Build history of the part. All positions in model axes, mm. A direction names the side the tool comes from. Give positions to 0.01 mm unless a question says otherwise; leave off trailing zeros. Loops run counter-clockwise (first coordinate to the right, second up) from the corner with the lowest first, then second, coordinate; pieces in that order, holes last. Notation, with made-up numbers: (6, 45.25) -> (20, 45.25) arc R36 ccw to (20, 80.25) -> close; hole circle Ø3 at (79.25, 22.25). An arc over 180 degrees is marked (long way). One line per question, with ' | ' between items. Start each with the question number.
(1) 3-axis set-ups, long thin cutter, end or side, ignore diameter. For faces 4 (the face through (92.284, 68.059, 113.109)), 5 (the face through (33.459, 79.964, 195.719)), 6 (the face through (105.51, 15.34, 49.21)): which of +Z, -Z, +X, -X, +Y, -Y reach the whole face in a straight line?
(2) Slice it at A-A, the plane z = 120.65. Write the cut outline in (x, y), then the cut area to 3 significant figures.
(3) Slice it at C-C, the plane z = 41.5. Write the cut outline in (x, y).
(4) Mould opens along X. For faces 1 (the face through (70.713, 79.585, 68.393)), 2 (the face through (-5.603, 19, 79)), 3 (the face through (104.887, 19, 79)) say: pulls with the +X half, pulls with the -X half, needs draft (parallel to the pull), parting line crosses it, or undercut.
(5) Slice it at D-D, the plane y = 15.24. Write the cut outline in (x, z).
(6) Drill centre lines: L1, parallel to X at y = 12, z = 105.5; L2, parallel to X at y = 72, z = 141; L3, parallel to Z at x = 105, y = 15. Where is each one in solid material? Low to high. Write a range as from..to.
(7) Flat gauge pins, fed straight in: pin 1 Ø1.4 at (x, z) = (105.5, 33.5) entering from -Y; pin 2 Ø0.6 at (x, z) = (-5, 30.5) entering from +Y; pin 3 Ø8 at (x, z) = (86, 138.5) entering from +Y; pin 4 Ø1.5 at (y, z) = (46.5, 153) entering from -X. Where does each tip first touch, or does it go through?
(8) Slice it at B-B, the plane y = 32. Write the cut outline in (x, z), then the cut area to 3 significant figures.
```python
from build123d import *

# Parameters (mm, degrees)
BOSS_EXTRUDE1_DEPTH = 196.85
CUT_EXTRUDE1_DEPTH  = 152.4
SKETCH3_R           = 4.7625
CUT_EXTRUDE2_DEPTH  = 152.4


with BuildPart() as part:
    # Sketch1 → Boss-Extrude1 (new body)
    with BuildSketch(Plane.XY):
        with BuildLine():
            Line((-5.602925898, 0), (-4.332925898, 0))
            Line((-4.332925898, 0), (-4.332925898, 38.1))
            ThreePointArc((-4.332925898, 38.1), (7.942228903, 67.7348452), (37.577074102, 80.01))
            Line((37.577074102, 80.01), (62.977074102, 80.01))
            ThreePointArc((62.977074102, 80.01), (92.611919302, 67.7348452), (104.887074102, 38.1))
            Line((104.887074102, 38.1), (104.887074102, 0))
            Line((104.887074102, 0), (106.157074102, 0))
            Line((106.157074102, 0), (106.157074102, 38.1))
            ThreePointArc((106.157074102, 38.1), (93.509944914, 68.632870812), (62.977074102, 81.28))
            Line((62.977074102, 81.28), (37.577074102, 81.28))
            ThreePointArc((37.577074102, 81.28), (7.04420329, 68.632870812), (-5.602925898, 38.1))
            Line((-5.602925898, 38.1), (-5.602925898, 0))
        make_face()
    extrude(amount=BOSS_EXTRUDE1_DEPTH)

    # Sketch2 → Cut-Extrude1 (cut)
    with BuildSketch(Plane.ZY.offset(5.602925898)):
        Polygon((0, 0), (69.85, 81.28), (0, 81.28), align=None)
        Polygon((196.85, 81.28), (127, 0), (196.85, 0), align=None)
    extrude(amount=-CUT_EXTRUDE1_DEPTH, mode=Mode.SUBTRACT)

    # Sketch3 → Cut-Extrude2 (cut)
    with BuildSketch(Plane.ZY.offset(5.602925898)):
        with Locations((120.65, 15.24)):
            Circle(SKETCH3_R)
        with BuildLine():
            Line((25.4, 20.0025), (44.45, 20.0025))
            ThreePointArc((44.45, 20.0025), (49.2125, 15.24), (44.45, 10.4775))
            Line((44.45, 10.4775), (25.4, 10.4775))
            ThreePointArc((25.4, 10.4775), (20.6375, 15.24), (25.4, 20.0025))
        make_face()
    extrude(amount=-CUT_EXTRUDE2_DEPTH, mode=Mode.SUBTRACT)


solid = part.part
```
Final values:
1) face 4: +Z, -Z, -Y | face 5: +Z, +X, -X, -Y | face 6: +X, -X
2) outline: (-5.6, 0) -> (-4.33, 0) -> (-4.33, 10.48) -> (-5.6, 10.48) -> close; (-5.6, 20) -> (-4.33, 20) -> (-4.33, 38.1) arc R41.91 cw to (37.58, 80.01) -> (62.98, 80.01) arc R41.91 cw to (104.89, 38.1) -> (104.89, 20) -> (106.16, 20) -> (106.16, 38.1) arc R43.18 ccw to (62.98, 81.28) -> (37.58, 81.28) arc R43.18 ccw to (-5.6, 38.1) -> close; (104.89, 0) -> (106.16, 0) -> (106.16, 10.48) -> (104.89, 10.48) -> close | area: 275 mm2
3) outline: (-5.6, 0) -> (-4.33, 0) -> (-4.33, 10.48) -> (-5.6, 10.48) -> close; (-5.6, 20) -> (-4.33, 20) -> (-4.33, 38.1) arc R41.91 cw to (-3.08, 48.29) -> (-4.38, 48.29) arc R43.18 ccw to (-5.6, 38.1) -> close; (103.63, 48.29) arc R41.91 cw to (104.89, 38.1) -> (104.89, 20) -> (106.16, 20) -> (106.16, 38.1) arc R43.18 ccw to (104.94, 48.29) -> close; (104.89, 0) -> (106.16, 0) -> (106.16, 10.48) -> (104.89, 10.48) -> close
4) face 1: needs draft | face 2: pulls with the -X half | face 3: undercut
5) outline: (-5.6, 13.1) -> (-4.33, 13.1) -> (-4.33, 20.64) -> (-5.6, 20.64) -> close; (-5.6, 49.21) -> (-4.33, 49.21) -> (-4.33, 115.89) -> (-5.6, 115.89) -> close; (-5.6, 125.41) -> (-4.33, 125.41) -> (-4.33, 140.1) -> (-5.6, 140.1) -> close; (104.89, 13.1) -> (106.16, 13.1) -> (106.16, 20.64) -> (104.89, 20.64) -> close; (104.89, 49.21) -> (106.16, 49.21) -> (106.16, 115.89) -> (104.89, 115.89) -> close; (104.89, 125.41) -> (106.16, 125.41) -> (106.16, 140.1) -> (104.89, 140.1) -> close
6) L1: -5.6..-4.33, 104.89..106.16 | L2: 10.83..12.93, 87.62..89.72 | L3: 12.89..20.64, 49.21..115.89, 125.41..139.89
7) pin 1: y = 0 | pin 2: y = 35.84 | pin 3: y = 76.86 | pin 4: x = -4.92
8) outline: (-5.6, 27.5) -> (-4.33, 27.5) -> (-4.33, 154.5) -> (-5.6, 154.5) -> close; (104.89, 27.5) -> (106.16, 27.5) -> (106.16, 154.5) -> (104.89, 154.5) -> close | area: 323 mm2
